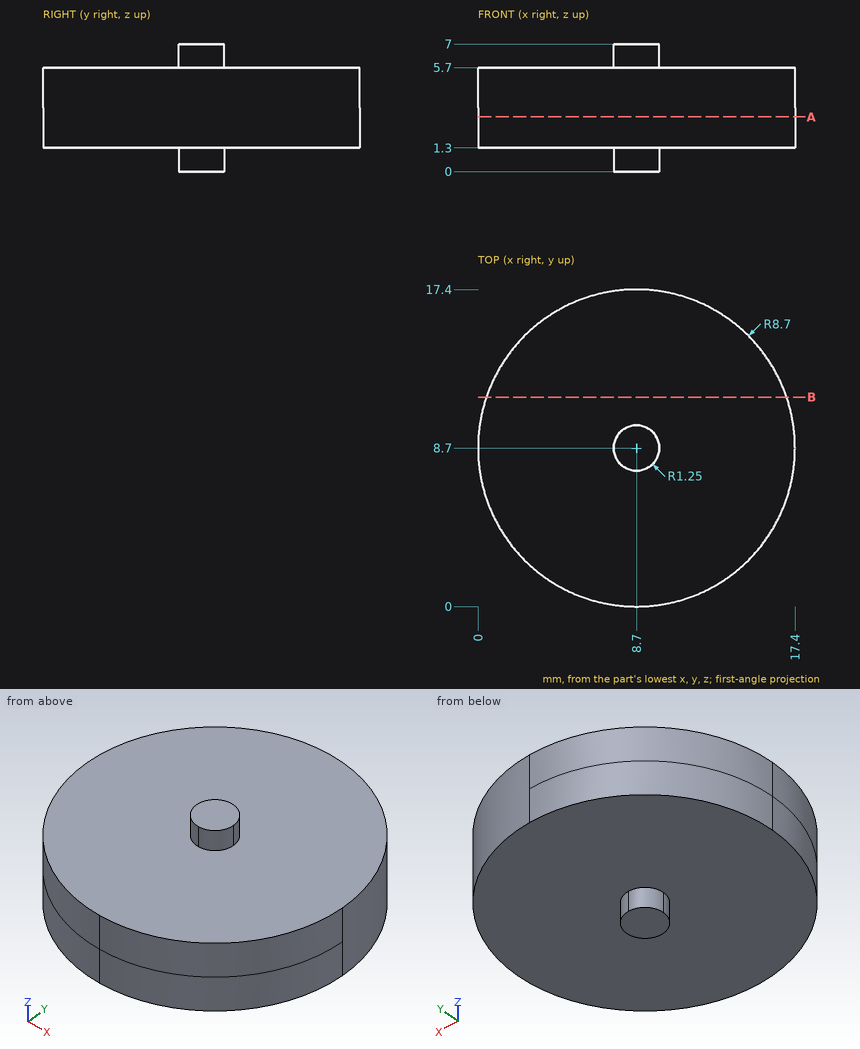
Could you check a few things on this drawing? It's one solid part, dimensions in mm from its lowest x, y, z. Give positions to 0.01 mm unless a question says otherwise; leave off trailing zeros. Loops run counter-clockwise (first coordinate to the right, second up) from the corner with the lowest first, then second, coordinate; pieces in that order, holes last. Notation, with made-up numbers: M 82.5,85 L 88.5,85 A26 cw 88.5,120 Z; hole C 16,-8.5 d3. An arc over 180 degrees is marked long. One line per question, with ' | ' between items. Start each with the question number.
Q1. If I drill on line 1 (Z direction, x = 11, y = 15.5); line 2 (X direction, y = 9, z = 2.25), over which ranges is the centre line in solid material (lowest first)? Write a range as from..to.
Q2. For pin 1 Ø1.5 at (x, y) = (12.5, 5) entering from -Z; pin 2 Ø1.5 at (x, y) = (12, 13.5) entering from +Z; pin 3 Ø2 at (y, z) = (10.5, 1.5) entering from -X, each with a flat end and sliding along its axis, tell me the tip position at first contact or that it passes through.
Q3. If we section it at A-A (z = 3): Please give me the cut outline in (x, y).
Q4. If we section it at B-B (y = 11.5): Please give me the cut outline in (x, z).
Computed:
1) line 1: z = 1.3..5.7 | line 2: x = 0.01..17.39
2) pin 1: stops at z = 1.3 | pin 2: stops at z = 5.7 | pin 3: stops at x = 0.04
3) outline: C 8.7,8.7 d17.4
4) outline: M 0.46,1.3 L 16.94,1.3 L 16.94,5.7 L 0.46,5.7 Z
